Geometry: final body of the model. Coordinates: model frame, mm. Face numbers are marked on the shaded views. Round coordinates to 2 decimals unless told otherwise and drop trailing zeros. Order: outer loops, then holes, each group sorted by start corner. A loop starts at its lowest first (then second) coordinate and runs counter-clockwise, first axis right, second up. Notation, with made-up numbers: M 61.5,47 L 87.5,47 A28 cw 87.5,68 Z; hole C -3,84.5 d6. An arc over 180 degrees is marked long. Put each result on its own line as item: value. Start each with the question number.
1) Draft query along Z for the marked faces 1 and 2. Return one class per face: pulls with the +Z half, pulls with the -Z half, needs draft (parallel to the pull), parting line crosses it, or undercut.
2) Section B-B, the plane x = -36. Return loops of the section in (y, z), then the cut area to 3 significant figures.
3) Section C-C, the plane y = 5. Return loops of the section in (x, z).
4) Section A-A, the plane z = 0.1. Return loops of the section in (x, y) (3 decimals), then the cut area to 3 significant figures.
5) Material intervals for probe 1 along Y at (x, z) = (50.8, 0.2) (3 decimals); probe 2 along X at (y, z) = (-27.5, 0.2), sorted ascending. Write a range as [from, to].
from build123d import *

# Parameters (mm, degrees)
SKETCH2_R           = 1.475
BOSS_EXTRUDE1_DEPTH = 0.254
FILLET1_R           = 6.35


with BuildPart() as part:
    # Sketch2 → Boss-Extrude1 (new body)
    # profile 1 of 3: a face of its own
    with BuildSketch(Plane.XY):
        with BuildLine():
            ThreePointArc((-6.35, -37.972720471), (-8.946176851, -37.446173633), (-11.5, -36.742346142))
            ThreePointArc((-11.5, -36.742346142), (-22.79802623, 31.024184115), (38.5, 0))
            ThreePointArc((38.5, 0), (31.024184115, -22.79802623), (11.5, -36.742346142))
            ThreePointArc((11.5, -36.742346142), (8.946176851, -37.446173633), (6.35, -37.972720471))
            Line((6.35, -37.972720471), (6.35, -44.45))
            Line((6.35, -44.45), (57.15, -44.45))
            Line((57.15, -44.45), (57.15, 44.45))
            Line((57.15, 44.45), (-57.15, 44.45))
            Line((-57.15, 44.45), (-57.15, -44.45))
            Line((-57.15, -44.45), (-6.35, -44.45))
            Line((-6.35, -44.45), (-6.35, -37.972720471))
        make_face()
        with Locations((-50.8, 0)):
            Circle(SKETCH2_R, mode=Mode.SUBTRACT)
        with Locations((50.8, 0)):
            Circle(SKETCH2_R, mode=Mode.SUBTRACT)
    # profile 2 of 3: a face of its own
    with BuildSketch(Plane.XY):
        with BuildLine():
            Line((11.5, -36.742346142), (6.35, -36.742346142))
            Line((6.35, -36.742346142), (6.35, -37.972720471))
            ThreePointArc((6.35, -37.972720471), (8.946176851, -37.446173633), (11.5, -36.742346142))
        make_face()
    # profile 3 of 3: a face of its own
    with BuildSketch(Plane.XY):
        with BuildLine():
            Line((-6.35, -36.742346142), (-11.5, -36.742346142))
            ThreePointArc((-11.5, -36.742346142), (-8.946176851, -37.446173633), (-6.35, -37.972720471))
            Line((-6.35, -37.972720471), (-6.35, -36.742346142))
        make_face()
    extrude(amount=BOSS_EXTRUDE1_DEPTH)

    # Fillet1
    fillet1_edges = [part.edges().sort_by_distance(p)[0] for p in [
        (-57.15, -44.45, 0.127),
        (-57.15, 44.45, 0.127),
        (57.15, 44.45, 0.127),
        (57.15, -44.45, 0.127),
    ]]
    fillet(fillet1_edges, radius=FILLET1_R)


solid = part.part
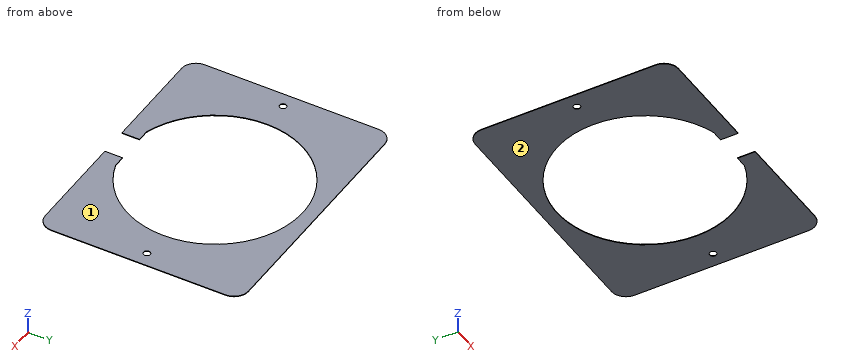
Result sheet:
1. face 1: pulls with the +Z half
1. face 2: pulls with the -Z half
2. outline: M -44.45,0 L -13.65,0 L -13.65,0.25 L -44.45,0.25 Z; M 13.65,0 L 44.45,0 L 44.45,0.25 L 13.65,0.25 Z
2. area: 15.6 mm2
3. outline: M -57.15,0 L -38.17,0 L -38.17,0.25 L -57.15,0.25 Z; M 38.17,0 L 57.15,0 L 57.15,0.25 L 38.17,0.25 Z
4. outline: M -57.15,-38.1 A6.35 ccw -50.8,-44.45 L -6.35,-44.45 L -6.35,-36.742 L -11.5,-36.742 A38.5 cw long 11.5,-36.742 L 6.35,-36.742 L 6.35,-44.45 L 50.8,-44.45 A6.35 ccw 57.15,-38.1 L 57.15,38.1 A6.35 ccw 50.8,44.45 L -50.8,44.45 A6.35 ccw -57.15,38.1 Z; hole C -50.8,0 d2.95; hole C 50.8,0 d2.95
4. area: 5,390 mm2
5. probe 1: y = [-44.45, -1.475], [1.475, 44.45]
5. probe 2: x = [-57.15, -26.94], [26.94, 57.15]
